```python
from build123d import *

# Parameters (mm, degrees)
F0_R     = 1.1811
F0_R_2   = 1.5875
F1_DEPTH = 0.8001


with BuildPart() as f1:
    # F0 (on Front) → F1 (new body, symmetric)
    with BuildSketch(Plane.XZ):
        with BuildLine():
            Line((5.280381, 3.991776), (-7.04344, 3.991776))
            ThreePointArc((-7.04344, 3.991776), (-3.637121, -4.925726), (5.280381, -1.519407))
            Line((5.280381, -1.519407), (5.280381, 3.991776))
        make_face()
        with Locations((-0.881529, -3.777536)):
            Circle(F0_R, mode=Mode.SUBTRACT)
        with Locations((-0.881529, 1.236185)):
            Circle(F0_R_2, mode=Mode.SUBTRACT)
    extrude(amount=F1_DEPTH, both=True)


solid = f1.part
```
Input: part model. Units: mm. Frame: model coordinates. Round coordinates to 2 decimals unless told otherwise and drop trailing zeros. Write each loop counter-clockwise with the first axis right and the second up, starting at its lowest first coordinate (ties: lowest second). Pieces come first, ordered by that corner, then holes. Notation, with made-up numbers: (59, -26.75) -> (114, -26.75) arc R28 cw to (114, -0.75) -> close; hole circle Ø10 at (57.25, -25.75). An arc over 180 degrees is marked (long way). Answer as CSV lines item,"result".
1. Section A-A (z = -4.5). Return the cut outline in (x, y), plus the area to 3 significant figures.
Geometry says:
outline,"(-4.44, -0.8) -> (-1.82, -0.8) -> (-1.82, 0.8) -> (-4.44, 0.8) -> close; (0.05, -0.8) -> (2.68, -0.8) -> (2.68, 0.8) -> (0.05, 0.8) -> close"
area,"8.40 mm^2"
2. Section C-C (z = 2). Return the cut outline in (x, y).
Geometry says:
outline,"(-7.59, -0.8) -> (-2.27, -0.8) -> (-2.27, 0.8) -> (-7.59, 0.8) -> close; (0.51, -0.8) -> (5.28, -0.8) -> (5.28, 0.8) -> (0.51, 0.8) -> close"
3. Section B-B (x = 0). Return the cut outline in (y, z), plus the area to 3 significant figures.
Geometry says:
outline,"(-0.8, -5.46) -> (0.8, -5.46) -> (0.8, -4.56) -> (-0.8, -4.56) -> close; (-0.8, -2.99) -> (0.8, -2.99) -> (0.8, -0.08) -> (-0.8, -0.08) -> close; (-0.8, 2.56) -> (0.8, 2.56) -> (0.8, 3.99) -> (-0.8, 3.99) -> close"
area,"8.38 mm^2"
4. Ray query, L1, parallel to Z at x = -1.5, y = 0.65; L2, parallel to Z at x = -0.75, y = -0.1; L3, parallel to X at y = -0.3, z = -3.5. Return the intervals inside material, ascending. Write a range as [from, to].
Geometry says:
L1,"z = [-5.49, -4.78], [-2.77, -0.23], [2.7, 3.99]"
L2,"z = [-5.51, -4.95], [-2.6, -0.35], [2.82, 3.99]"
L3,"x = [-5.69, -2.03], [0.27, 3.93]"
5. Section D-D (y = -0.4). Give the number of separate pieces and of enclosed holes in the cut face, plus the area to 3 significant figures.
Geometry says:
separate pieces,"1"
enclosed holes,"2"
area,"93.2 mm^2"
6. Mould query, pull axis X, two halves, no side actions, for faces 1 (the cylindrical face through (0.21, 0.01, -4.23)), 2 (the flat face through (-1, -0.8, -1)), 3 (the cylindrical face through (-3.772, -0.011, -4.864)). Classes: +X half, -X half, draft (parallel to the pull), parting line (faces both ways), or undercut.
Geometry says:
face 1,"undercut"
face 2,"draft"
face 3,"parting line"
